Answer from the drawing. Dimensions are ordinates in mm from the lowest x, y and z of the part. A direction names the side the tool comes from. Give positions to 0.01 mm unless a question says otherwise; leave off trailing zeros. Loops run counter-clockwise (first coordinate to the right, second up) from the corner with the lowest first, then second, coordinate; pieces in that order, holes last. Notation, with made-up numbers: (73, 54) - (80, 54) arc R8 cw to (80, 63) - close; hole circle Ø5 at (88.5, 10.5). An arc over 180 degrees is marked (long way). One line per item, written item: value.
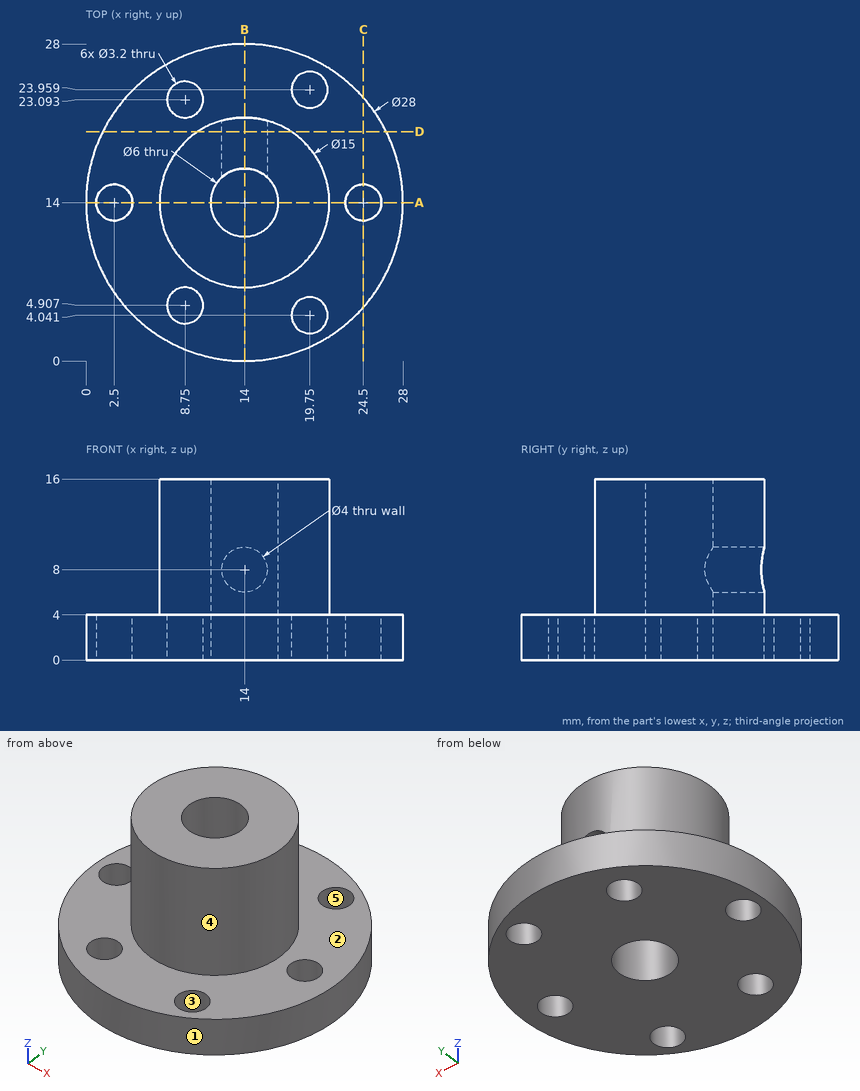
1. Section C-C (x = 24.5) is taken. Write down the section's boundary in (y, z), and give its area (3 significant figures).
Output:
outline: (4.74, 0) - (12.4, 0) - (12.4, 4) - (4.74, 4) - close; (15.6, 0) - (23.26, 0) - (23.26, 4) - (15.6, 4) - close
area: 61.3 mm²
2. For the marked faces 4 and 5, determine the directions among +Z, -Z, +X, -X, +Y, -Y from which every point of the face is accessible in a straight line to the end or side of a thin tool.
Output:
face 4: +Z
face 5: +Z, -Z
3. Section D-D (y = 20.25) is taken. Write down the section's boundary in (x, z).
Output:
outline: (1.47, 0) - (26.53, 0) - (26.53, 4) - (18.15, 4) - (18.15, 16) - (9.85, 16) - (9.85, 4) - (1.47, 4) - close; hole circle Ø4 at (14, 8)
4. Section A-A (y = 14) is taken. Write down the section's boundary in (x, z).
Output:
outline: (0, 0) - (0.9, 0) - (0.9, 4) - (0, 4) - close; (4.1, 0) - (11, 0) - (11, 16) - (6.5, 16) - (6.5, 4) - (4.1, 4) - close; (17, 0) - (22.9, 0) - (22.9, 4) - (21.5, 4) - (21.5, 16) - (17, 16) - close; (26.1, 0) - (28, 0) - (28, 4) - (26.1, 4) - close
5. Flat-ended cylindrical pins translate along their axes: pin 1 Ø6 at (y, z) = (18, 11) entering from +X; pin 2 Ø1.5 at (y, z) = (24.5, 2.5) entering from +X; pin 3 Ø5 at (x, y) = (24.5, 14) entering from +Z. Find the tip coordinate at first contact, or state that the pin passes through.
Output:
pin 1: stops at x = 21.43
pin 2: stops at x = 24.05
pin 3: stops at z = 4
6. The mould has two halves that part along X. Classify the marked faces 1, 2 and 3: released by +X, released by -X, zero draft, split by the parting line, or undercut.
Output:
face 1: split by the parting line
face 2: zero draft
face 3: undercut
7. Find the intervals of material crossed by line 1 along X through (y, z) = (14, 5.25); line 2 along Y through (x, z) = (19.75, 2.8) (1 decimal); line 3 along Y through (x, z) = (19, 2.5) (1 decimal), in increasing order.
Output:
line 1: x = 6.5 to 11, 17 to 21.5
line 2: y = 1.2 to 2.4, 5.6 to 22.4, 25.6 to 26.8
line 3: y = 0.9 to 2.6, 5.5 to 22.5, 25.4 to 27.1
8. Section B-B (x = 14) is taken. Write down the section's boundary in (y, z), and give its area (3 significant figures).
Output:
outline: (0, 0) - (11, 0) - (11, 16) - (6.5, 16) - (6.5, 4) - (0, 4) - close; (17, 0) - (28, 0) - (28, 4) - (21.5, 4) - (21.5, 6) - (17, 6) - close; (17, 10) - (21.5, 10) - (21.5, 16) - (17, 16) - close
area: 178 mm²
